Here's how the part is built. I have some questions about the finished solid (model axes, mm). Give positions to 0.01 mm unless a question says otherwise; leave off trailing zeros. Order: outer loops, then holes, each group sorted by start corner. A loop starts at its lowest first (then second) coordinate and runs counter-clockwise, first axis right, second up. Notation, with made-up numbers: M 64.5,-13.5 L 97.5,-13.5 A33 ccw 97.5,16.5 Z; hole C 29,63.5 d6. An arc over 180 degrees is marked long. One line per item, written item: value. Start each with the question number.
from build123d import *

# Parameters (mm, degrees)
SKETCH_1_R          = 200
EXTRUDE_1_DEPTH     = 3
SKETCH_2_R          = 10
CUT_EXTRUDE_1_DEPTH = 3
SKETCH_3_W          = 60
SKETCH_3_H          = 60
CUT_EXTRUDE_2_DEPTH = 3


with BuildPart() as part:
    # 草图1 → 凸台-拉伸1 (new body)
    with BuildSketch(Plane(origin=(0, 0, 0), x_dir=(1, 0, 0), z_dir=(0, 1, 0))):
        with Locations(Location((0, 0, 0), (0, 0, 270))):
            Circle(SKETCH_1_R)
    extrude(amount=EXTRUDE_1_DEPTH)

    # 草图2 → 切除-拉伸1 (cut)
    with BuildSketch(Plane(origin=(0, 3, 0), x_dir=(1, 0, 0), z_dir=(0, 1, 0))):
        with Locations(Location((-113.13708499, 113.13708499, 0), (0, 0, 270))):
            Circle(SKETCH_2_R)
        with Locations(Location((-113.13708499, -113.13708499, 0), (0, 0, 90))):
            Circle(SKETCH_2_R)
        with Locations(Location((113.13708499, -113.13708499, 0), (0, 0, 270))):
            Circle(SKETCH_2_R)
        with Locations(Location((113.13708499, 113.13708499, 0), (0, 0, 90))):
            Circle(SKETCH_2_R)
    extrude(amount=-CUT_EXTRUDE_1_DEPTH, mode=Mode.SUBTRACT)

    # 草图3 → 切除-拉伸2 (cut)
    with BuildSketch(Plane(origin=(0, 3, 0), x_dir=(1, 0, 0), z_dir=(0, 1, 0))):
        Rectangle(SKETCH_3_W, SKETCH_3_H)
    extrude(amount=-CUT_EXTRUDE_2_DEPTH, mode=Mode.SUBTRACT)


solid = part.part
Item 1: I want a section at B-B on x = 0. Write out the boundary of the cut face in (y, z).
Item 2: Will these pins go through, and if not, where does the flat tip stop? P1, Ø1.5, axis at y = 2.5, z = 89, coming from the -X side; P2, Ø1, axis at x = -104.5, z = 61, coming from the -Y side; P3, Ø1, axis at y = 2.5, z = -81.5, coming from the +X side.
Item 3: I want a section at D-D on z = -116. Write out the boundary of the cut face in (x, y), plus the area to 3 significant figures.
Item 4: I want a section at C-C on y = 0.7. Write out the boundary of the cut face in (x, z), plus the area to 3 significant figures.
Item 5: We'd pull the mould along Z, two halves only. Please class faces 1 (the face through (123.052, 1.521, 111.835)), 2 (the face through (-42, 3, -3)), 3 (the face through (103.22, 1.52, -111.84)), 4 (the face through (60.075, 1.479, 190.764)): +Z half, -Z half, draft (parallel to the pull), parting line (faces both ways), or undercut.
Item 6: I want a section at A-A on z = 0. Write out the boundary of the cut face in (x, y).
Item 7: Please list where these lines run through material, in increasing order: probe 1 along Z at (x, y) = (-121, 1.05); probe 2 along X at (y, z) = (1.3, 107.5); probe 3 along X at (y, z) = (2.05, 111). Write a range as [from, to].
Answer below:
1. outline: M 0,-200 L 3,-200 L 3,-30 L 0,-30 Z; M 0,30 L 3,30 L 3,200 L 0,200 Z
2. P1: stops at x = -179.48
2. P2: stops at y = 0
2. P3: stops at x = 182.86
3. outline: M -162.92,0 L -122.72,0 L -122.72,3 L -162.92,3 Z; M -103.56,0 L 103.56,0 L 103.56,3 L -103.56,3 Z; M 122.72,0 L 162.92,0 L 162.92,3 L 122.72,3 Z
3. area: 863 mm²
4. outline: C 0,0 d400; hole C -113.14,-113.14 d20; hole C -113.14,113.14 d20; hole M -30,-30 L 30,-30 L 30,30 L -30,30 Z; hole C 113.14,-113.14 d20; hole C 113.14,113.14 d20
4. area: 121,000 mm²
5. face 1: undercut
5. face 2: draft
5. face 3: undercut
5. face 4: parting line
6. outline: M -200,0 L -30,0 L -30,3 L -200,3 Z; M 30,0 L 200,0 L 200,3 L 30,3 Z
7. probe 1: z = [-159.25, -119.32], [-106.96, 106.96], [119.32, 159.25]
7. probe 2: x = [-168.65, -121.4], [-104.88, 104.88], [121.4, 168.65]
7. probe 3: x = [-166.37, -122.91], [-103.37, 103.37], [122.91, 166.37]
